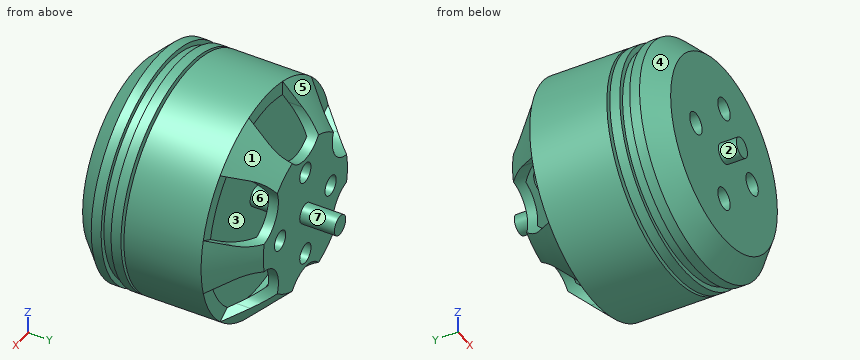
```python
from build123d import *

# Parameters (mm, degrees)
SKETCH4_R          = 1.1
CUT_EXTRUDE1_DEPTH = 3.5
SKETCH5_R          = 1
CUT_EXTRUDE2_DEPTH = 4


with BuildPart() as part:
    # Sketch2 → Revolve1 (revolve)
    with BuildSketch(Plane.XY):
        Polygon((0, 0), (-1, 0), (-1, -22.38), (0, -22.38), (0, -20.58), (8.5, -20.58), (10.5, -18.58), (10.5, -17.58), (10, -17.58), (10, -16.58), (10.5, -16.58), (10.5, -15.58), (8.5, -15.58), (8.5, -15.28), (10.5, -15.28), (10.5, -7.5), (6.5, -3.5), (0, -3.5), align=None)
        Polygon((1, -4.5), (6.085786438, -4.5), (9.5, -7.914213562), (9.5, -8.5), (0, -8.5), (0, -5.5), (1, -5.5), align=None, mode=Mode.SUBTRACT)
    revolve(axis=Axis((-1, 0, 0), (0, -1, 0)))

    # Sketch4 → Cut-Extrude1 (cut)
    with BuildSketch(Plane.XZ.offset(20.58)):
        with Locations((-1, 5)):
            Circle(SKETCH4_R)
        with Locations((4, 0)):
            Circle(SKETCH4_R)
        with Locations((-1, -5)):
            Circle(SKETCH4_R)
        with Locations((-6, 0)):
            Circle(SKETCH4_R)
    extrude(amount=-CUT_EXTRUDE1_DEPTH, mode=Mode.SUBTRACT)

    # Sketch5 → Cut-Extrude2 (cut)
    with BuildSketch(Plane(origin=(0, -3.5, 0), x_dir=(1, 0, 0), z_dir=(0, 1, 0))):
        with Locations((-1, 4.5)):
            Circle(SKETCH5_R)
        with Locations((3.5, 0)):
            Circle(SKETCH5_R)
        with Locations((-1, -4.5)):
            Circle(SKETCH5_R)
        with Locations((-5.5, 0)):
            Circle(SKETCH5_R)
        with BuildLine():
            Line((2, 9), (2, 12))
            Line((2, 12), (-4, 12))
            Line((-4, 12), (-4, 9))
            ThreePointArc((-4, 9), (-1, 6), (2, 9))
        make_face()
        with BuildLine():
            Line((8.294228634, 1.901923789), (10.892304845, 3.401923789))
            Line((10.892304845, 3.401923789), (7.892304845, 8.598076211))
            Line((7.892304845, 8.598076211), (5.294228634, 7.098076211))
            ThreePointArc((5.294228634, 7.098076211), (4.196152423, 3), (8.294228634, 1.901923789))
        make_face()
        with BuildLine():
            Line((5.294228634, -7.098076211), (7.892304845, -8.598076211))
            Line((7.892304845, -8.598076211), (10.892304845, -3.401923789))
            Line((10.892304845, -3.401923789), (8.294228634, -1.901923789))
            ThreePointArc((8.294228634, -1.901923789), (4.196152423, -3), (5.294228634, -7.098076211))
        make_face()
        with BuildLine():
            Line((-4, -9), (-4, -12))
            Line((-4, -12), (2, -12))
            Line((2, -12), (2, -9))
            ThreePointArc((2, -9), (-1, -6), (-4, -9))
        make_face()
        with BuildLine():
            Line((-10.294228634, -1.901923789), (-12.892304845, -3.401923789))
            Line((-12.892304845, -3.401923789), (-9.892304845, -8.598076211))
            Line((-9.892304845, -8.598076211), (-7.294228634, -7.098076211))
            ThreePointArc((-7.294228634, -7.098076211), (-6.196152423, -3), (-10.294228634, -1.901923789))
        make_face()
        with BuildLine():
            Line((-7.294228634, 7.098076211), (-9.892304845, 8.598076211))
            Line((-9.892304845, 8.598076211), (-12.892304845, 3.401923789))
            Line((-12.892304845, 3.401923789), (-10.294228634, 1.901923789))
            ThreePointArc((-10.294228634, 1.901923789), (-6.196152423, 3), (-7.294228634, 7.098076211))
        make_face()
    extrude(amount=-CUT_EXTRUDE2_DEPTH, mode=Mode.SUBTRACT)


solid = part.part
```
Could you check a few things on this model? Use its own coordinates, in mm. Face numbers are marked on the shaded views. A direction names the side the tool comes from. Coordinates: 2 decimals unless noted, no trailing zeros. Loops run counter-clockwise (first coordinate to the right, second up) from the corner with the lowest first, then second, coordinate; pieces in that order, holes last.
1) Which directions (+Z, -Z, +X, -X, +Y, -Y) give clear straight access to the entire face, cutting with the end or side of a thin tool? Please do the marked faces 5, 6 and 7.
Reported:
face 5: +Z, -X, +Y
face 6: none
face 7: +Y
2) Thinking about a two-plate mould opening in Y: for the marked faces 1, 2, 3 and 4, which applies, released by +Y, released by -Y, zero draft, split by the parting line, or undercut?
Reported:
face 1: released by +Y
face 2: zero draft
face 3: undercut
face 4: released by -Y
3) Imagine slicing it at A-A (x = -1). State how many separate pieces and enclosed holes the cut face has, and give its area (3 significant figures).
Reported:
separate pieces: 3
enclosed holes: 0
area: 287 mm2
4) Will these pins go through, and if not, where does the flat tip stop? pin 1 Ø4.5 at (x, z) = (-10, 5) entering from +Y; pin 2 Ø10 at (y, z) = (-13, 8.5) entering from +X; pin 3 Ø1.5 at (y, z) = (-20, -4.5) entering from +X.
Reported:
pin 1: stops at y = -7.5
pin 2: stops at x = 9.95
pin 3: stops at x = 8.92
5) Imagine slicing it at C-C (y = -16). List the corners of the cut face in (x, z) for me, and give its area (3 significant figures).
Reported:
outline: circle Ø23 at (-1, 0)
area: 415 mm2
6) Please list where these lines run through material, in increasing order: line 1 along Y through (x, z) = (-2.75, 6.5); line 2 along Y through (x, z) = (4.5, 8.75); line 3 along Z through (x, y) = (-1, -18.6).
Reported:
line 1: y = -20.58 to -8.5, -4.5 to -3.5
line 2: y = -19.74 to -15.58, -15.28 to -8.5, -7.75 to -6.34
line 3: z = -11.48 to -6.1, -3.9 to 3.9, 6.1 to 11.48
